from build123d import *

# Parameters (mm, degrees)
F0_W     = 13
F0_H     = 44
F1_DEPTH = 25.4


with BuildPart() as f1:
    # F0 (on Top) → F1 (new body)
    with BuildSketch(Plane.XY):
        Polygon((33, 20.5), (33, 70.5), (-68, 70.5), (-68, -70.5), (-28.3125, -70.5), (-28.3125, -30.5), (-15.3125, -30.5), (-15.3125, -70.5), (68, -70.5), (68, 20.5), align=None)
        with Locations((-22.5, 42.5)):
            Rectangle(F0_W, F0_H, mode=Mode.SUBTRACT)
    extrude(amount=F1_DEPTH)


solid = f1.part
Verification items for the finished model (mm, model axes). A direction names the side the tool comes from. Give positions to 0.01 mm unless a question says otherwise; leave off trailing zeros. Loops run counter-clockwise (first coordinate to the right, second up) from the corner with the lowest first, then second, coordinate; pieces in that order, holes last.
1) Depth check by flat-ended pin: pin 1 Ø7.5 at (x, z) = (52.5, 9) entering from +Y; pin 2 Ø10.5 at (x, z) = (-21.5, 18.5) entering from -Y; pin 3 Ø1 at (x, y) = (12, -33.5) entering from -Z; pin 4 Ø12.5 at (y, z) = (38, 10) entering from +X. Enter the tip coordinate at first touch or a pass-through.
2) Draft check along Y on faces 1 (the flat face through (-29, 42, 13)), 2 (the flat face through (-17, 70.5, 13)), 3 (the flat face through (33, 45, 13)). Enter one of: pulls with the +Y half, pulls with the -Y half, needs draft (parallel to the pull), parting line crosses it, or undercut.
3) Thickness scan on line 1 along X through (y, z) = (-49, 20.75); line 2 along X through (y, z) = (56.5, 5.5); line 3 along Y through (x, z) = (49.5, 8.5). Record the ranges inside material, lowest first.
4) Sectioned sample at A-A, the plane y = 28. Enter the section's corners in (x, z), then the cut area to 3 significant figures.
5) Set-up check for faces 4 (the flat face through (-15.312, -50, 13)), 5 (the flat face through (-16, 42, 13)), 6 (the flat face through (51, 20.5, 13)): record each of +Z, -Z, +X, -X, +Y, -Y from which the full face is reachable in a straight line by a thin tool's end or side.
6) Sectioned sample at B-B, the plane z = 21.5. Enter the section's corners in (x, y), then the cut area to 3 significant figures.
Answers:
1. pin 1: stops at y = 20.5
1. pin 2: stops at y = -30.5
1. pin 3: stops at z = 0
1. pin 4: stops at x = 33
2. face 1: undercut
2. face 2: pulls with the +Y half
2. face 3: needs draft
3. line 1: x = -68 to -28.31, -15.31 to 68
3. line 2: x = -68 to -29, -16 to 33
3. line 3: y = -70.5 to 20.5
4. outline: (-68, 0) - (-29, 0) - (-29, 25.4) - (-68, 25.4) - close; (-16, 0) - (33, 0) - (33, 25.4) - (-16, 25.4) - close
4. area: 2,240 mm2
5. face 4: +Z, -Z, -Y
5. face 5: +Z, -Z
5. face 6: +Z, -Z, +X, +Y
6. outline: (-68, -70.5) - (-28.31, -70.5) - (-28.31, -30.5) - (-15.31, -30.5) - (-15.31, -70.5) - (68, -70.5) - (68, 20.5) - (33, 20.5) - (33, 70.5) - (-68, 70.5) - close; hole (-29, 20.5) - (-16, 20.5) - (-16, 64.5) - (-29, 64.5) - close
6. area: 16,300 mm2
